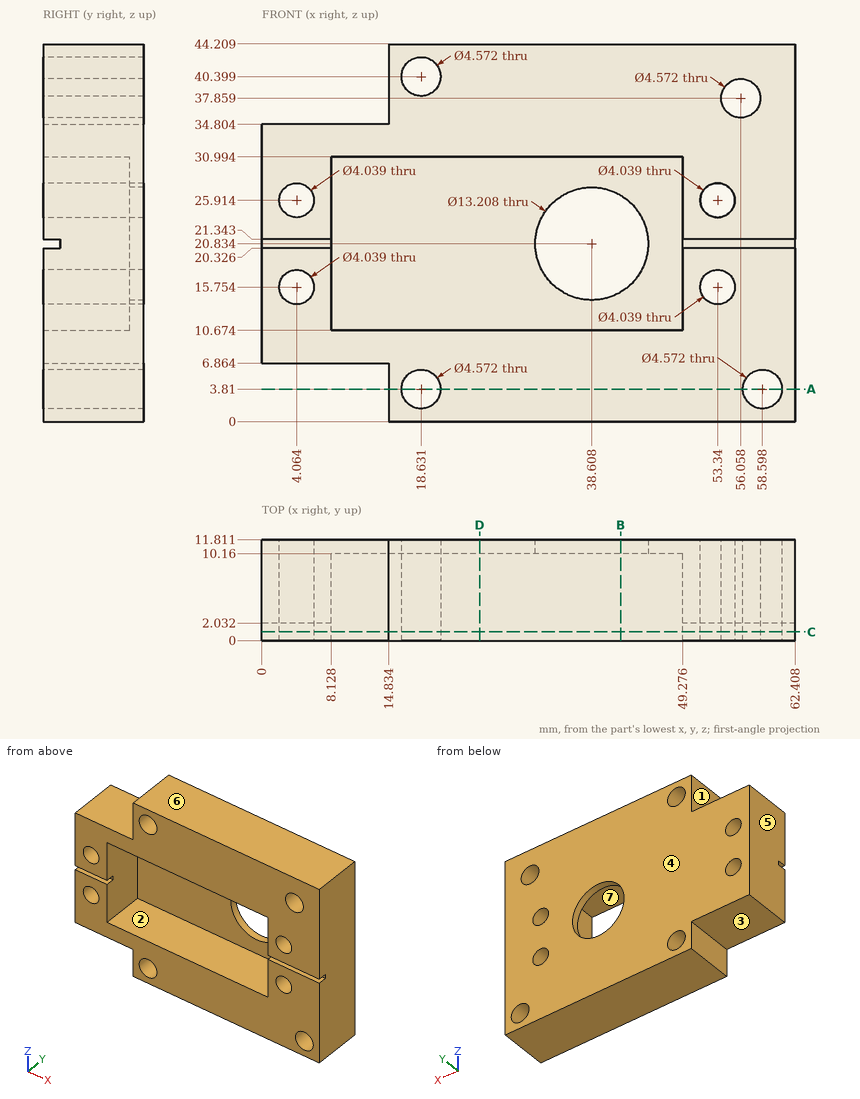
Part print with two shaded views. Sizes in mm from the minimum x, y, z corner. A direction names the side the tool comes from. Coordinates: 2 decimals unless noted, no trailing zeros. Loops run counter-clockwise (first coordinate to the right, second up) from the corner with the lowest first, then second, coordinate; pieces in that order, holes last. Notation, with made-up numbers: (26, -28) - (67, -28) arc R13 cw to (67, -10) - close; hole circle Ø9 at (72, -29). An arc over 180 degrees is marked (long way). Write each question's results on one line, items separated by ' | '. Start each with the question number.
Q1. Slice it at B-B on x = 42. Give the cut face in (y, z) (1 decimal), and give its area (3 significant figures).
Q2. Slice it at C-C on y = 1. Give the number of separate pieces and of enclosed holes in the cut face, and give its area (3 significant figures).
Q3. Two-plate mould, pull along X, no slides. Class the marked faces 5, 6 and 7: +X half, -X half, draft (parallel to the pull), parting line (faces both ways), or undercut.
Q4. Probe line 1 along Z through (x, y) = (53.34, 5.5) (1 decimal); line 2 along Z through (x, y) = (28.5, 4.25) (1 decimal); line 3 along X through (y, z) = (3.5, 28.5) (1 decimal). List the from-to ranges inside material, lowest first.
Q5. Which spindle directions (+Z, -Z, +X, -X, +Y, -Y) get a long thin tool onto all of the face, cutting with end or side? Do the marked faces 1, 2, 3 and 4. Say none if no direction does.
Q6. Drop flat-ended pins along their axis: pin 1 Ø1.6 at (x, y) = (3, 1) entering from -Z (1 decimal); pin 2 Ø6 at (x, z) = (23, 21.5) entering from -Y; pin 3 Ø0.5 at (x, z) = (2.5, 21) entering from -Y. Give the stop position or say it passes through.
Q7. Slice it at D-D on x = 25.5. Give the cut face in (y, z) (1 decimal).
Q8. Slice it at A-A on z = 3.81. Give the cut face in (x, y) (1 decimal).
Answer:
1) outline: (0, 0) - (11.8, 0) - (11.8, 15.2) - (10.2, 15.2) - (10.2, 10.7) - (0, 10.7) - close; (0, 31) - (10.2, 31) - (10.2, 26.5) - (11.8, 26.5) - (11.8, 44.2) - (0, 44.2) - close | area: 297 mm2
2) separate pieces: 2 | enclosed holes: 8 | area: 1,540 mm2
3) face 5: -X half | face 6: draft | face 7: undercut
4) line 1: z = 0 to 13.7, 17.8 to 23.9, 27.9 to 44.2 | line 2: z = 0 to 10.7, 31 to 44.2 | line 3: x = 0 to 8.1, 49.3 to 62.4
5) face 1: +Z, -X, +Y, -Y | face 2: -Y | face 3: -Z, -X, +Y, -Y | face 4: +Z, -Z, +X, -X, +Y
6) pin 1: stops at z = 6.9 | pin 2: stops at y = 10.16 | pin 3: stops at y = 2.03
7) outline: (0, 0) - (11.8, 0) - (11.8, 44.2) - (0, 44.2) - (0, 31) - (10.2, 31) - (10.2, 10.7) - (0, 10.7) - close
8) outline: (14.8, 0) - (16.3, 0) - (16.3, 11.8) - (14.8, 11.8) - close; (20.9, 0) - (56.3, 0) - (56.3, 11.8) - (20.9, 11.8) - close; (60.9, 0) - (62.4, 0) - (62.4, 11.8) - (60.9, 11.8) - close
